Source: three-view drawing plus pictorial views. Frame: mm from the lowest corner of the part. A direction names the side the tool comes from. Round coordinates to 2 decimals unless told otherwise and drop trailing zeros. Loops run counter-clockwise (first coordinate to the right, second up) from the corner with the lowest first, then second, coordinate; pieces in that order, holes last. Notation, with made-up numbers: (22, 81.25) -> (38, 81.25) arc R24 cw to (38, 108.25) -> close; hole circle Ø1 at (46, 17). An arc over 180 degrees is marked (long way). Answer in a Markdown table with one row per item.
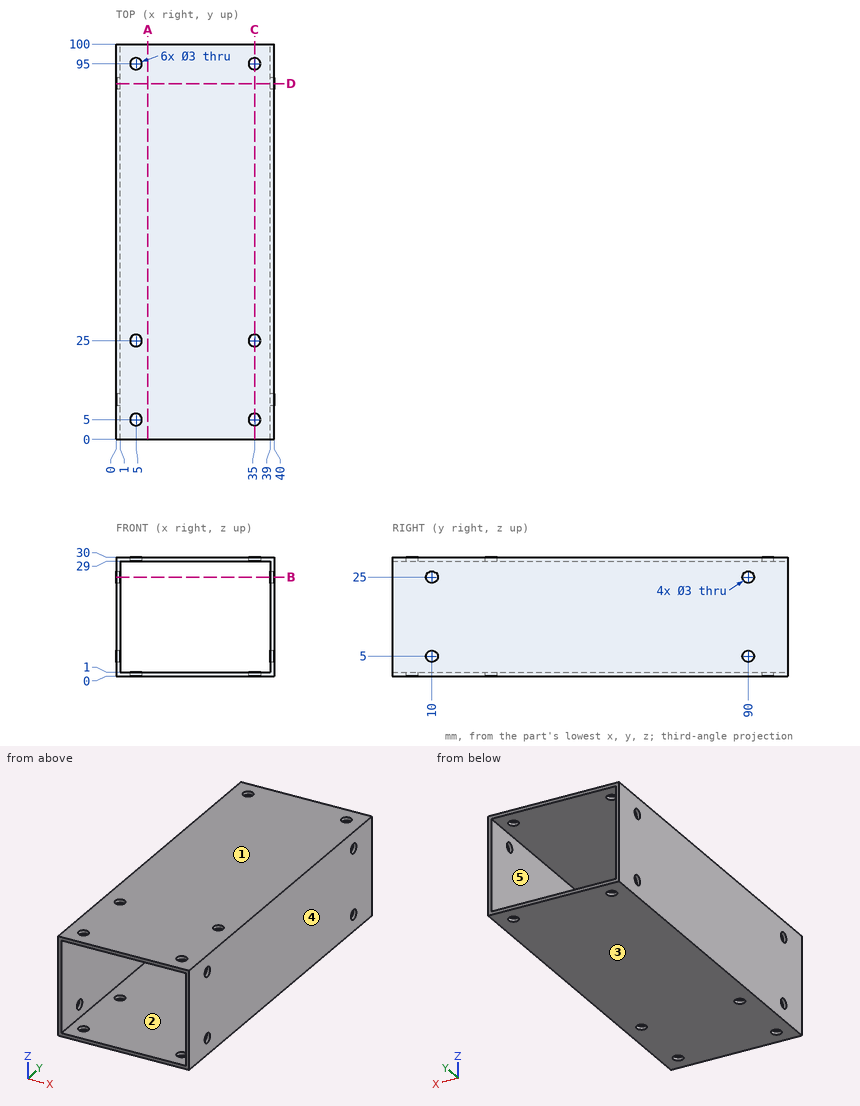
Item 1: Cut plane D-D (y = 90). Output: boundary loops of the cut face in (x, z), then the cut area to 3 significant figures.
Answer:
| item | result |
|---|---|
| outline | (0, 0) -> (40, 0) -> (40, 3.5) -> (39, 3.5) -> (39, 1) -> (1, 1) -> (1, 3.5) -> (0, 3.5) -> close; (0, 6.5) -> (1, 6.5) -> (1, 23.5) -> (0, 23.5) -> close; (0, 26.5) -> (1, 26.5) -> (1, 29) -> (39, 29) -> (39, 26.5) -> (40, 26.5) -> (40, 30) -> (0, 30) -> close; (39, 6.5) -> (40, 6.5) -> (40, 23.5) -> (39, 23.5) -> close |
| area | 124 mm² |
Item 2: Line query: probe 1 along Y at (x, z) = (5, 0.45); probe 2 along Z at (x, y) = (0.5, 90); probe 3 along X at (y, z) = (12, 12.5). Output: solid intervals per line, ascending. Write a range as [from, to].
Answer:
| item | result |
|---|---|
| probe 1 | y = [0, 3.5], [6.5, 23.5], [26.5, 93.5], [96.5, 100] |
| probe 2 | z = [0, 3.5], [6.5, 23.5], [26.5, 30] |
| probe 3 | x = [0, 1], [39, 40] |
Item 3: Draft query along Z for the marked faces 3, 4 and 5. Return one class per face: pulls with the +Z half, pulls with the -Z half, needs draft (parallel to the pull), parting line crosses it, or undercut.
Answer:
| item | result |
|---|---|
| face 3 | pulls with the -Z half |
| face 4 | needs draft |
| face 5 | undercut |
Item 4: Cut plane C-C (x = 35). Count the separate pieces of the cut face and the enclosed holes in it, then the cut area to 3 significant figures.
Answer:
| item | result |
|---|---|
| separate pieces | 8 |
| enclosed holes | 0 |
| area | 182 mm² |
Item 5: Cut plane A-A (x = 8). Output: boundary loops of the cut face in (y, z).
Answer:
| item | result |
|---|---|
| outline | (0, 0) -> (100, 0) -> (100, 1) -> (0, 1) -> close; (0, 29) -> (100, 29) -> (100, 30) -> (0, 30) -> close |
Item 6: Cut plane B-B (z = 25). Output: boundary loops of the cut face in (x, y).
Answer:
| item | result |
|---|---|
| outline | (0, 0) -> (1, 0) -> (1, 8.5) -> (0, 8.5) -> close; (0, 11.5) -> (1, 11.5) -> (1, 88.5) -> (0, 88.5) -> close; (0, 91.5) -> (1, 91.5) -> (1, 100) -> (0, 100) -> close; (39, 0) -> (40, 0) -> (40, 8.5) -> (39, 8.5) -> close; (39, 11.5) -> (40, 11.5) -> (40, 88.5) -> (39, 88.5) -> close; (39, 91.5) -> (40, 91.5) -> (40, 100) -> (39, 100) -> close |
Item 7: Reachability of the marked faces 1 and 2 from +Z, -Z, +X, -X, +Y, -Y: full face, straight path, thin tool, end or side. Return the list, or none.
Answer:
| item | result |
|---|---|
| face 1 | +Z, +X, -X, +Y, -Y |
| face 2 | +Y, -Y |
